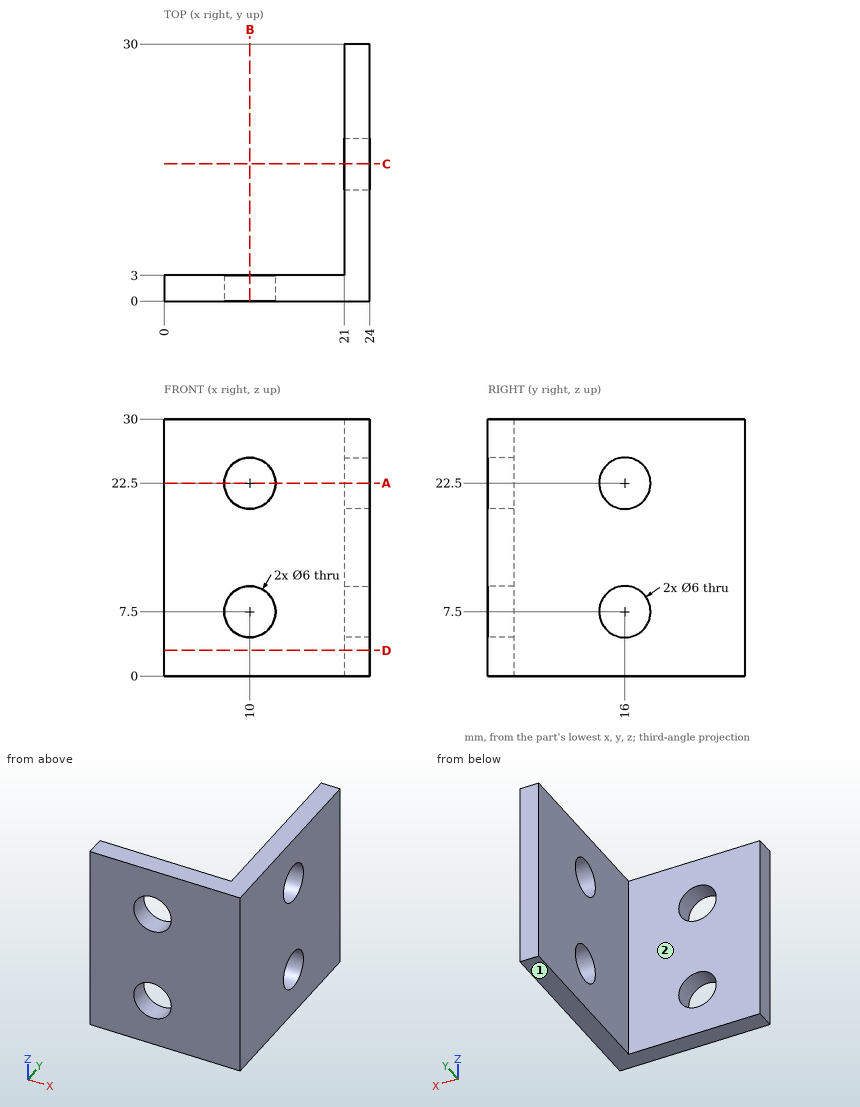
Study the drawing (mm; zero at the part's minimum x, y, z) and answer. A direction names the side the tool comes from. Give positions to 0.01 mm unless a question says otherwise; leave off trailing zeros. Loops run counter-clockwise (first coordinate to the right, second up) from the corner with the lowest first, then second, coordinate; pieces in that order, holes last. Notation, with made-up numbers: M -4.75,-23.5 L 5.25,-23.5 A22 ccw 5.25,-15.5 Z; hole C 26,12.25 d9. An arc over 180 degrees is marked long. One line per item, written item: value. Start each with the question number.
1. Find section A-A (z = 22.5). Give the vertices of the cut face in (x, y), and give its area (3 significant figures).
2. Each of these flat-tipped pins is pushed along its axis until it touches: P1, Ø1.5, axis at x = 8.5, z = 26, coming from the +Y side; P2, Ø8, axis at y = 17, z = 14.5, coming from the -X side. Where does it stop, or does it pass through?
3. Find section C-C (y = 16). Give the vertices of the cut face in (x, z).
4. Find section D-D (z = 3). Give the vertices of the cut face in (x, y).
5. Which of the six approach directions +Z, -Z, +X, -X, +Y, -Y give full straight-line access (tool end or side, diameter ignored) to the marked faces 1 and 2?
6. Find the intervals of material crossed by probe 1 along Z at (x, y) = (10, 1.8); probe 2 along Y at (x, z) = (22.45, 22.5); probe 3 along Y at (x, z) = (12.5, 16.5), in increasing order.
7. Find section B-B (x = 10). Give the vertices of the cut face in (y, z).
Reported:
1. outline: M 0,0 L 7,0 L 7,3 L 0,3 Z; M 13,0 L 24,0 L 24,13 L 21,13 L 21,3 L 13,3 Z; M 21,19 L 24,19 L 24,30 L 21,30 Z
1. area: 117 mm²
2. P1: stops at y = 3
2. P2: stops at x = 21
3. outline: M 21,0 L 24,0 L 24,4.5 L 21,4.5 Z; M 21,10.5 L 24,10.5 L 24,19.5 L 21,19.5 Z; M 21,25.5 L 24,25.5 L 24,30 L 21,30 Z
4. outline: M 0,0 L 24,0 L 24,30 L 21,30 L 21,3 L 0,3 Z
5. face 1: -Z, +X, -X, +Y, -Y
5. face 2: +Z, -Z, -X, +Y
6. probe 1: z = 0 to 4.5, 10.5 to 19.5, 25.5 to 30
6. probe 2: y = 0 to 13, 19 to 30
6. probe 3: y = 0 to 3
7. outline: M 0,0 L 3,0 L 3,4.5 L 0,4.5 Z; M 0,10.5 L 3,10.5 L 3,19.5 L 0,19.5 Z; M 0,25.5 L 3,25.5 L 3,30 L 0,30 Z
